Here's how the part is built. I have some questions about the finished solid (model axes, mm). Round coordinates to 2 decimals unless told otherwise and drop trailing zeros. Order: outer loops, then holes, each group sorted by start corner. A loop starts at its lowest first (then second) coordinate and runs counter-clockwise, first axis right, second up. Notation, with made-up numbers: M -10,-23 L 33,-23 A23 cw 33,16 Z; hole C -25,83.5 d3. An arc over 180 degrees is marked long. Write item = value, one per line. Start each with the question number.
Item 1: I want a section at B-B, the plane x = -20. State how many separate pieces and enclosed holes the cut face has, plus the area to 3 significant figures.
Item 2: I'm going to push a flat-ended pin straight in: P1, Ø1, axis at y = 17, z = 4.5, coming from the -X side. Where does the tip first touch, or does it pass through?
Item 3: I want a section at A-A, the plane y = 20. List the corners of the cut face in (x, z) for me.
Item 4: Please list where these lines run through material, in increasing order: L1, parallel to Y at x = 19, z = 1; L2, parallel to Z at x = -13, y = 10.
Autodesk Inventor part; units mm, degrees
ref_plane "YZ Plane" through (0, 0, 0) normal (1, 0, 0) x (0, 1, 0)
ref_plane "XZ Plane" through (0, 0, 0) normal (0, 1, 0) x (-1, 0, 0)
ref_plane "XY Plane" through (0, 0, 0) normal (0, 0, 1) x (1, 0, 0)
ref_plane "Arbeitsebene1" through (0, 0, 0) normal (0, 0, 1) x (1, 0, 0)
sketch "Skizze1" plane through (0, 0, 0) normal (0, 0, 1) x (1, 0, 0)
  arc A0 (-22.9, 24.9) -> (-24.9, 22.9) centre (-22.9, 22.9) ccw
  line L0 (-24.9, 22.9) -> (-24.9, -22.9)
  arc A1 (-24.9, -22.9) -> (-22.9, -24.9) centre (-22.9, -22.9) ccw
  line L1 (-22.9, -24.9) -> (22.9, -24.9)
  arc A2 (22.9, -24.9) -> (24.9, -22.9) centre (22.9, -22.9) ccw
  line L2 (24.9, -22.9) -> (24.9, 22.9)
  arc A3 (24.9, 22.9) -> (22.9, 24.9) centre (22.9, 22.9) ccw
  line L3 (22.9, 24.9) -> (-22.9, 24.9)
  circle A4 centre (20, 20) radius 1.6
  circle A5 centre (-20, -20) radius 1.6
  circle A6 centre (20, -20) radius 1.6
  circle A7 centre (-20, 20) radius 1.6
  arc A8 (6.7383, -21.066) -> (8.3017, -21.066) centre (7.52, -20.62) ccw
  line L4 (6.7383, -21.066) -> (-6.9383, -21.066)
  arc A9 (-8.5017, -21.066) -> (-6.9383, -21.066) centre (-7.72, -20.62) ccw
  line L5 (-8.5017, -21.066) -> (-17.9, -21.066)
  line L6 (-17.9, -21.066) -> (-17.9, 21.066)
  line L7 (-17.9, 21.066) -> (17.9, 21.066)
  line L8 (17.9, 21.066) -> (17.9, 12)
  arc A10 (14.9, 9) -> (17.9, 12) centre (14.9, 12) ccw
  line L9 (14.5, 9) -> (14.9, 9)
  arc A11 (14.5, 9) -> (11.5, 6) centre (14.5, 6) ccw
  line L10 (11.5, -6) -> (11.5, 6)
  arc A12 (11.5, -6) -> (14.5, -9) centre (14.5, -6) ccw
  line L11 (14.9, -9) -> (14.5, -9)
  arc A13 (17.9, -12) -> (14.9, -9) centre (14.9, -12) ccw
  line L12 (17.9, -12) -> (17.9, -21.066)
  line L13 (17.9, -21.066) -> (8.3017, -21.066)
  arc A14 (13.4381, 5.6873) -> (13.3881, 5.2) centre (15.7881, 5.2) ccw
  line L14 (13.4381, 5.6873) -> (13.4381, 7.6)
  line L15 (13.4381, 7.6) -> (15.7881, 7.6)
  arc A15 (18.1881, 5.2) -> (15.7881, 7.6) centre (15.7881, 5.2) ccw
  line L16 (18.1881, 5.2) -> (18.1881, -5.2)
  arc A16 (15.7881, -7.6) -> (18.1881, -5.2) centre (15.7881, -5.2) ccw
  line L17 (15.7881, -7.6) -> (13.4381, -7.6)
  line L18 (13.4381, -7.6) -> (13.4381, -5.6873)
  arc A17 (13.3881, -5.2) -> (13.4381, -5.6873) centre (15.7881, -5.2) ccw
  line L19 (13.3881, -5.2) -> (13.3881, 5.2)
  line L20 (17.9, 21.066) -> (17.9, -21.066)
  point P0 (0, 0)
extrude "Extrusion1" add sketch "Skizze1" along normal blind 7 contours L3 A3 L2 A2 L1 A1 L0 A0 | A4 | A5 | A6 | A7 | L4 A9 L5 L6 L7 L8 A10 L9 A11 L10 A12 L11 A13 L12 L13 A8 | A13 L11 A12 L10 A11 L9 A10 L20 A15 L15 L14 A14 L19 A17 L18 L17 A16 | L20 A15 L16 A16 | A16 L17 L18 A17 L19 A14 L14 L15 A15 L20
sketch "Skizze2" plane through (0, 0, 7) normal (0, 0, 1) x (1, 0, 0)
  circle A0 centre (-20, 20) radius 1.6
  circle A1 centre (20, 20) radius 1.6
  circle A2 centre (20, -20) radius 1.6
  circle A3 centre (-20, -20) radius 1.6
  line L0 (24.9, -22.9) -> (24.9, 22.9)
  line L1 (-24.9, 0.75) -> (24.9, 0.75)
  line L2 (24.9, 0.75) -> (24.9, -0.75)
  line L3 (24.9, -0.75) -> (-24.9, -0.75)
  line L4 (-24.9, -0.75) -> (-24.9, 0.75)
  line L5 (-24.9, 0.75) -> (24.9, -0.75) construction
  line L6 (24.9, 0.75) -> (-24.9, -0.75) construction
  point P0 (0, 0)
  dimension "d2" = 1.5
extrude "Extrusion2" cut sketch "Skizze2" against normal blind 5.5 contours L3 L4 L1 L0
pattern_linear "Rechteckige Anordnung1" count 10 spacing 2.5 along (0, -1, 0) count 10 spacing 2.5 along (0, 1, 0) of "Extrusion2"
sketch "Skizze3" plane through (0, 0, 7) normal (0, 0, 1) x (1, 0, 0)
  circle A0 centre (-20, -20) radius 1.6
  line L0 (18.8686, -21.1314) -> (18.4, -21.6)
  arc A1 (22.9, -19.2319) -> (19.2319, -22.9) centre (20, -20) ccw
  circle A2 centre (20, 20) radius 1.6
  circle A3 centre (-20, 20) radius 1.6
  point P0 (0, 0)
hole "Bohrung1" at (-20, 20, 7) at (20, 20, 7) at (20, -20, 7) at (-20, -20, 7) direction (0, 0, -1) diameter 2.7 end through all
properties part number "10_Cube_sampleholder"
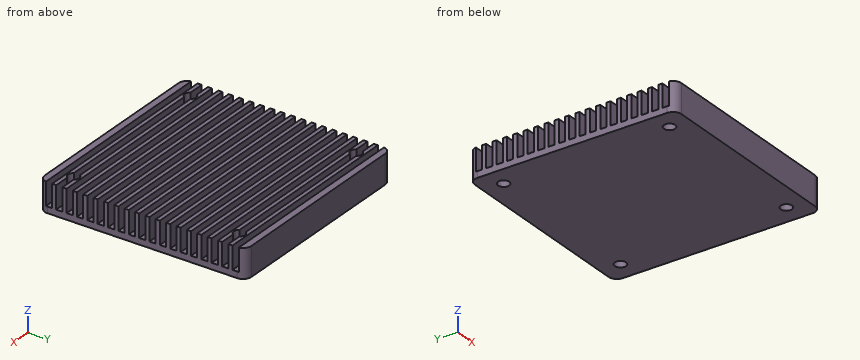
Filled in:
q1.separate_pieces = 3
q1.enclosed_holes = 0
q1.area = 171 mm^2
q2.P1 = -24.9
q3.outline = M -24.9,0 L -21.35,0 L -21.35,1.5 L -24.9,1.5 Z; M -18.65,0 L 18.65,0 L 18.65,1.5 L -18.65,1.5 Z; M 21.35,0 L 24.9,0 L 24.9,1.5 L 21.35,1.5 Z
q4.L1 = -24.9 to -20.91, -19.09 to 19.09, 20.91 to 24.9
q4.L2 = 0 to 1.5
